Part model, mm, in its own coordinate system. A direction names the side the tool comes from. Give positions to 0.01 mm unless a question says otherwise; leave off trailing zeros. Loops run counter-clockwise (first coordinate to the right, second up) from the corner with the lowest first, then second, coordinate; pieces in that order, holes last. Notation, with made-up numbers: M 59.25,-36 L 73.25,-36 A22 ccw 73.25,-20 Z; hole C 13,-39 d10. An arc over 180 degrees is marked long. Put each result on its own line as item: value. Start each with the question number.
```python
from build123d import *

# Parameters (mm, degrees)
SKETCH_1_R          = 1.5
EXTRUDE_1_DEPTH     = 2
SKETCH_2_R          = 0.5
CUT_EXTRUDE_1_DEPTH = 10
FILLET_2_R          = 1


with BuildPart() as part:
    # 草图1 → 凸台-拉伸1 (new body)
    with BuildSketch(Plane.XY):
        Polygon((15, -35), (15, -5.1), (4.9, -5.1), (4.9, 11.1), (25, 11.1), (25, 21), (-40, 21), (-40, 11.1), (-24.9, 11.1), (-24.9, 4.9), (-40, 4.9), (-40, -10.492736163), (-5, -35), align=None)
        with Locations((-35, 16)):
            Circle(SKETCH_1_R, mode=Mode.SUBTRACT)
        with Locations((10, -30)):
            Circle(SKETCH_1_R, mode=Mode.SUBTRACT)
        with Locations((10, -20)):
            Circle(SKETCH_1_R, mode=Mode.SUBTRACT)
        with Locations((0, 16)):
            Circle(SKETCH_1_R, mode=Mode.SUBTRACT)
        with Locations((20, 16)):
            Circle(SKETCH_1_R, mode=Mode.SUBTRACT)
        with Locations((-25, 0)):
            Circle(SKETCH_1_R, mode=Mode.SUBTRACT)
        Circle(SKETCH_1_R, mode=Mode.SUBTRACT)
        with Locations((0, -20)):
            Circle(SKETCH_1_R, mode=Mode.SUBTRACT)
        with Locations((0, -30)):
            Circle(SKETCH_1_R, mode=Mode.SUBTRACT)
    extrude(amount=EXTRUDE_1_DEPTH)

    # 草图2 → 切除-拉伸1 (cut)
    with BuildSketch(Plane(origin=(0, 0, 0), x_dir=(-1, 0, 0), z_dir=(0, 0, -1))):
        with Locations((-4.9, 11.1)):
            Circle(SKETCH_2_R)
        with Locations((-4.9, -5.1)):
            Circle(SKETCH_2_R)
        with Locations((24.9, 11.1)):
            Circle(SKETCH_2_R)
        with Locations((24.9, 4.9)):
            Circle(SKETCH_2_R)
    extrude(amount=-CUT_EXTRUDE_1_DEPTH, mode=Mode.SUBTRACT)

    # 圆角2
    fillet_2_edges = [part.edges().sort_by_distance(p)[0] for p in [
        (-40, 11.1, 1),
        (-40, 21, 1),
        (25, 21, 1),
        (25, 11.1, 1),
        (15, -5.1, 1),
        (15, -35, 1),
        (-5, -35, 1),
        (-40, -10.492736163, 1),
        (-40, 4.9, 1),
    ]]
    fillet(fillet_2_edges, radius=FILLET_2_R)


solid = part.part
```
1) Wall check: L1, parallel to Y at x = 0, z = 1.05; L2, parallel to X at y = 17, z = 1.4; L3, parallel to Y at x = -34.5, z = 1.5. Give the ranges that are in metal, low to high.
2) Band-saw the part on C-C on z = 1.7. State how many separate pieces and enclosed holes the cut face has, then the cut area to 3 significant figures.
3) Mould opens along Y. For faces 4 (the cylindrical face through (-0.195, -18.513, 0.986)), 5 (the flat face through (-8, -7, 2)), 6 (the flat face through (5, -35, 1)) say: +Y half, -Y half, draft (parallel to the pull), parting line (faces both ways), or undercut.
4) Band-saw the part on B-B on y = 0. Give the cut face in (x, z), then the cut area to 3 significant figures.
5) Which spindle directions (+Z, -Z, +X, -X, +Y, -Y) get a long thin tool onto all of the face, cutting with end or side? Do faces 1 (the flat face through (15, 11.1, 1)), 2 (the flat face through (15, -20, 1)), 3 (the flat face through (-32, 4.9, 1)). Say none if no direction does.
6) Pin check, flat tips, straight feed: pin 1 Ø1 at (y, z) = (-22, 1.5) entering from +X; pin 2 Ø1 at (y, z) = (10.5, 1) entering from -X. Stop position of each tip, or through.
7) Band-saw the part on D-D on y = 7.5. Give the cut face in (x, z).
8) Band-saw the part on A-A on x = 10. Give the cut face in (y, z), then the cut area to 3 significant figures.
Evaluation:
1. L1: -35 to -31.5, -28.5 to -21.5, -18.5 to -1.5, 1.5 to 14.5, 17.5 to 21
1. L2: -40 to -36.12, -33.88 to -1.12, 1.12 to 18.88, 21.12 to 25
1. L3: -14.34 to 4.9, 11.1 to 14.59, 17.41 to 21
2. separate pieces: 1
2. enclosed holes: 9
2. area: 2,430 mm2
3. face 4: undercut
3. face 5: draft
3. face 6: -Y half
4. outline: M -40,0 L -26.5,0 L -26.5,2 L -40,2 Z; M -23.5,0 L -1.5,0 L -1.5,2 L -23.5,2 Z; M 1.5,0 L 4.9,0 L 4.9,2 L 1.5,2 Z
4. area: 77.8 mm2
5. face 1: +Z, -Z, +X
5. face 2: +Z, -Z, +X, -Y
5. face 3: +Z, -Z, -X
6. pin 1: x = 15
6. pin 2: x = -24.9
7. outline: M -24.9,0 L 4.9,0 L 4.9,2 L -24.9,2 Z
8. outline: M -35,0 L -31.5,0 L -31.5,2 L -35,2 Z; M -28.5,0 L -21.5,0 L -21.5,2 L -28.5,2 Z; M -18.5,0 L -5.1,0 L -5.1,2 L -18.5,2 Z; M 11.1,0 L 21,0 L 21,2 L 11.1,2 Z
8. area: 67.6 mm2
